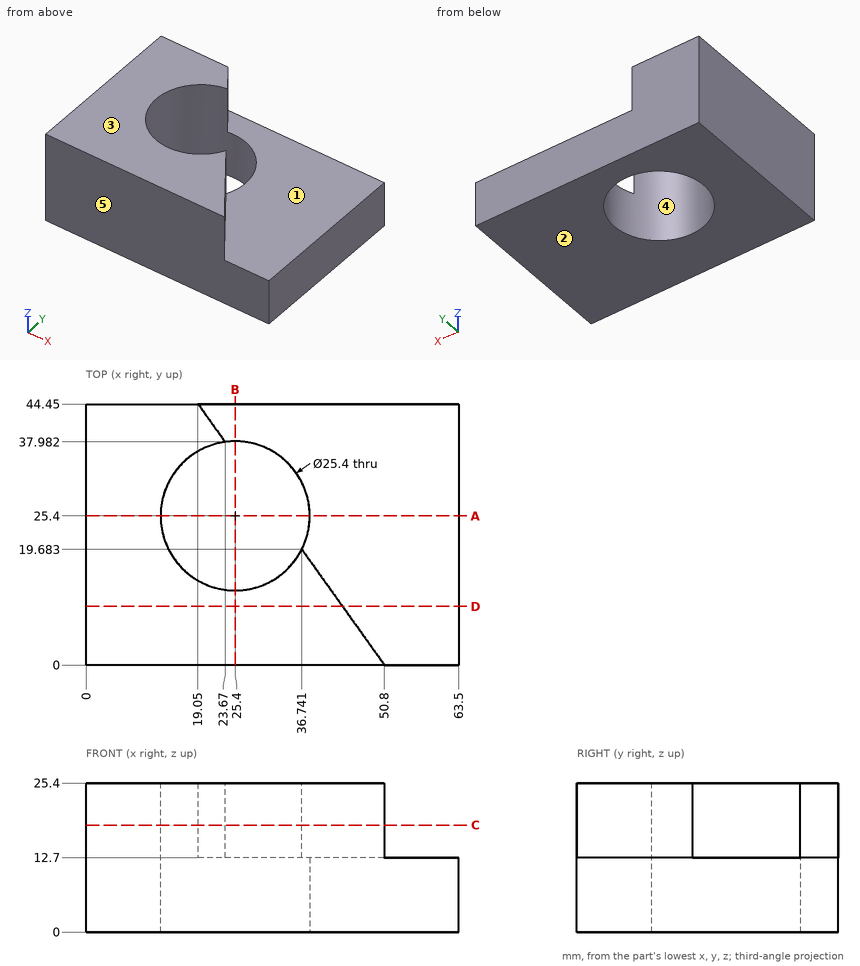
Answer from the drawing. Dimensions are ordinates in mm from the lowest x, y and z of the part. A direction names the side the tool comes from. Give positions to 0.01 mm unless a question says otherwise; leave off trailing zeros. Loops run counter-clockwise (first coordinate to the right, second up) from the corner with the lowest first, then second, coordinate; pieces in that order, holes last.
Item 1: The part is cut by section C-C (z = 18.25). Write down the section's boundary in (x, y).
Item 2: The part is cut by section A-A (y = 25.4). Write down the section's boundary in (x, z), and give its area (3 significant figures).
Item 3: The part is cut by section D-D (y = 10). Write down the section's boundary in (x, z), and give its area (3 significant figures).
Item 4: The mould has two halves that part along Y. Classify the marked faces 3, 4 and 5: released by +Y, released by -Y, zero draft, split by the parting line, or undercut.
Item 5: Find the intervals of material crossed by line 1 along Y through (x, z) = (25.4, 9.75); line 2 along Z through (x, y) = (40, 22.5); line 3 along X through (y, z) = (17, 24) (1 decimal), in increasing order.
Item 6: Each of these flat-tipped pins is pushed along its axis until it touches: pin 1 Ø4 at (x, z) = (44.5, 23) entering from +Y; pin 2 Ø1 at (y, z) = (19.5, 16.5) entering from +X. Where does it stop, or does it pass through?
Item 7: The part is cut by section B-B (x = 25.4). Write down the section's boundary in (y, z).
Item 8: For the marked faces 1 and 2, determine the directions among +Z, -Z, +X, -X, +Y, -Y from which every point of the face is accessible in a straight line to the end or side of a thin tool.
Taken from the geometry:
1. outline: (0, 0) - (50.8, 0) - (36.74, 19.68) arc R12.7 cw (long way) to (23.67, 37.98) - (19.05, 44.45) - (0, 44.45) - close
2. outline: (0, 0) - (12.7, 0) - (12.7, 25.4) - (0, 25.4) - close; (38.1, 0) - (63.5, 0) - (63.5, 12.7) - (38.1, 12.7) - close
2. area: 645 mm2
3. outline: (0, 0) - (63.5, 0) - (63.5, 12.7) - (43.66, 12.7) - (43.66, 25.4) - (0, 25.4) - close
3. area: 1,360 mm2
4. face 3: zero draft
4. face 4: undercut
4. face 5: released by -Y
5. line 1: y = 0 to 12.7, 38.1 to 44.45
5. line 2: z = 0 to 12.7
5. line 3: x = 0 to 15.9, 34.9 to 38.7
6. pin 1: stops at y = 11.62
6. pin 2: stops at x = 37.23
7. outline: (0, 0) - (12.7, 0) - (12.7, 25.4) - (0, 25.4) - close; (38.1, 0) - (44.45, 0) - (44.45, 12.7) - (38.1, 12.7) - close
8. face 1: +Z, +X, +Y
8. face 2: -Z, +X, -X, +Y, -Y
